Autodesk Fusion 360 part; units mm, degrees
sketch "Sketch1" plane through (0, 0, 0) normal (0, 0, 1) x (1, 0, 0)
  line L0 (-27.8831, 24.1702) -> (-27.8831, -24.1098)
  circle A0 centre (23.6169, -23.5198) radius 2.2
  arc A1 (24.2069, -27.9198) -> (28.0169, -24.1098) centre (24.2069, -24.1098) ccw
  line L1 (-24.0731, -27.9198) -> (24.2069, -27.9198)
  circle A2 centre (23.6169, 23.5802) radius 2.2
  line L2 (24.2069, 27.9802) -> (-24.0731, 27.9802)
  spline S0 degree 5 poles (28.0169, -21.3028) (28.0169, -21.1603) (28.0055, -20.8859) (27.9539, -20.5067) (27.8203, -20.0644) (27.5661, -19.6103) (27.2491, -19.2452) (26.8901, -18.9576) (26.4983, -18.7351) (26.0664, -18.5646) (25.5813, -18.4304) (25.0343, -18.3121) (24.4296, -18.1826) (23.7979, -18.0051) (23.1967, -17.7339) (22.6942, -17.3216) (22.4247, -16.8443) (22.3203, -16.389) (22.2971, -16.0405) (22.2971, -15.8549) knots -1 -1 -1 -1 -1 -1 -0.933333 -0.866667 -0.8 -0.733333 -0.666667 -0.6 -0.533333 -0.466667 -0.4 -0.333333 -0.266667 -0.2 -0.133333 -0.066667 0 0 0 0 0 0
  circle A3 centre (-23.4831, 23.5802) radius 2.2
  arc A4 (25.9741, -8.0941) -> (28.0169, -5.6032) centre (25.4769, -5.6032) ccw
  arc A5 (25.9741, -8.0941) -> (22.2971, -12.5777) centre (26.8691, -12.5777) ccw
  circle A6 centre (0.0669, 0.0302) radius 17.5
  arc A7 (-24.0731, 27.9802) -> (-27.8831, 24.1702) centre (-24.0731, 24.1702) ccw
  line L3 (22.2971, -15.8549) -> (22.2971, -12.5777)
  arc A8 (28.0169, 24.1702) -> (24.2069, 27.9802) centre (24.2069, 24.1702) ccw
  line L4 (28.0169, -5.6032) -> (28.0169, 24.1702)
  circle A9 centre (-23.4831, -23.5198) radius 2.2
  arc A10 (-27.8831, -24.1098) -> (-24.0731, -27.9198) centre (-24.0731, -24.1098) ccw
  line L5 (28.0169, -24.1098) -> (28.0169, -21.3028)
  circle A11 centre (-15.4271, 15.5242) radius 2.032
  circle A12 centre (15.5609, 15.5242) radius 2.032
  circle A13 centre (15.5609, -15.4638) radius 2.032
  circle A14 centre (-15.4271, -15.4638) radius 2.032
  circle A15 centre (-15.4271, -15.4638) radius 4.064
  circle A16 centre (15.5609, -15.4638) radius 4.064
  circle A17 centre (15.5609, 15.5242) radius 4.064
  circle A18 centre (-15.4271, 15.5242) radius 4.064
  dimension "d1" = 4.064
  dimension "d2" = 4.064
  dimension "d3" = 4.064
  dimension "d4" = 4.064
  dimension "d7" = 8.128
  dimension "d8" = 8.128
  dimension "d9" = 8.128
  dimension "d10" = 8.128
extrude "Extrude1" add sketch "Sketch1" along normal blind 11.684 contours L0 A1 L1 L2 S0 A4 A5 A7 L3 A8 L4 A10 L5 | A15 | A16 | A17 | A18
extrude "Extrude2" cut sketch "Sketch1" along normal blind 3.556 contours A15 | A16 | A17 | A18
Could you check a few things on this model? Use its own coordinates, in mm. A direction names the side the tool comes from. Give positions to 0.01 mm unless a question says otherwise; leave off trailing zeros. Write each loop counter-clockwise with the first axis right and the second up, starting at its lowest first coordinate (ties: lowest second). Pieces come first, ordered by that corner, then holes. Notation, with made-up numbers: (0.25, 89.5) -> (35.25, 89.5) arc R18 ccw to (35.25, 108.5) -> close; hole circle Ø7 at (-27.75, 52.25). An arc over 180 degrees is marked (long way). Answer as CSV lines item,"result". Start each with the question number.
(1) If we section it at B-B, the plane x = -3: Write out the boundary of the cut face in (y, z).
(2) If we mould it in two halves opening along X, with no side actions, what happens to faces 1 (the face through (0, -27.92, 6)), 2 (the face through (-27.883, 0, 6)), 3 (the face through (-13.24, -18.89, 1.75)), 4 (the face through (14.063, 14.151, 7.563))? For each: +X half, -X half, draft (parallel to the pull), parting line (faces both ways), or undercut.
(3) Please list where these lines run through material, in increasing order: line 1 (X direction, y = 23.5, z = 10); line 2 (Y direction, x = 25.5, z = 1.75); line 3 (Y direction, x = 15, z = 6).
(4) If we section it at A-A, the plane y = -2: Write out the boundary of the cut face in (x, z), and give its area (3 significant figures).
(5) Which directions (+Z, -Z, +X, -X, +Y, -Y) give clear straight access to the entire face, cutting with the end or side of a thin tool? Please do faces 5 (the face through (28.017, 9, 6)), 6 (the face through (23.31, -9.71, 5.76)), 7 (the face through (17.3, -17.2, 3.556)).
(6) If we section it at C-C, the plane y = -22.5: Write out the boundary of the cut face in (x, z), and give its area (3 significant figures).
(7) If we section it at D-D, the plane x = 14.5: Write out the boundary of the cut face in (y, z).
(8) I'm going to push flat-ended pins straight in: pin 1 Ø3.5 at (y, z) = (-13.5, 5) entering from +X; pin 2 Ø5 at (x, y) = (15.56, 15.52) entering from -Z. Where does each tip first touch, or does it pass through?
Answer list:
1,outline,"(-27.92, 0) -> (-17.2, 0) -> (-17.2, 11.68) -> (-27.92, 11.68) -> close; (17.26, 0) -> (27.98, 0) -> (27.98, 11.68) -> (17.26, 11.68) -> close"
2,face 1,"draft"
2,face 2,"-X half"
2,face 3,"undercut"
2,face 4,"undercut"
3,line 1,"-27.88 to -25.68, -21.28 to 21.42, 25.82 to 28.02"
3,line 2,"-27.69 to -24.66, -22.38 to -18.42, -8.22 to 22.44, 24.72 to 27.75"
3,line 3,"-27.92 to -17.42, -13.51 to -9.09, 9.15 to 13.57, 17.48 to 27.98"
4,outline,"(-27.88, 0) -> (-17.31, 0) -> (-17.31, 11.68) -> (-27.88, 11.68) -> close; (17.45, 0) -> (28.02, 0) -> (28.02, 11.68) -> (17.45, 11.68) -> close"
4,area,"247 mm^2"
5,face 5,"+Z, -Z, +X, +Y, -Y"
5,face 6,"+Z, -Z, +X"
5,face 7,"-Z"
6,outline,"(-27.88, 0) -> (-25.43, 0) -> (-25.43, 11.68) -> (-27.88, 11.68) -> close; (-21.53, 0) -> (21.67, 0) -> (21.67, 11.68) -> (-21.53, 11.68) -> close; (25.57, 0) -> (28.02, 0) -> (28.02, 11.68) -> (25.57, 11.68) -> close"
6,area,"562 mm^2"
7,outline,"(-27.92, 0) -> (-19.39, 0) -> (-19.39, 3.56) -> (-17.2, 3.56) -> (-17.2, 11.68) -> (-27.92, 11.68) -> close; (-13.73, 3.56) -> (-11.54, 3.56) -> (-11.54, 0) -> (-9.87, 0) -> (-9.87, 11.68) -> (-13.73, 11.68) -> close; (9.93, 0) -> (11.6, 0) -> (11.6, 3.56) -> (13.79, 3.56) -> (13.79, 11.68) -> (9.93, 11.68) -> close; (17.26, 3.56) -> (19.45, 3.56) -> (19.45, 0) -> (27.98, 0) -> (27.98, 11.68) -> (17.26, 11.68) -> close"
8,pin 1,"x = 22.37"
8,pin 2,"z = 3.56"
